Autodesk Inventor part; units mm, degrees
ref_plane "YZ Plane" through (0, 0, 0) normal (1, 0, 0) x (0, 1, 0)
ref_plane "XZ Plane" through (0, 0, 0) normal (0, 1, 0) x (-1, 0, 0)
ref_plane "XY Plane" through (0, 0, 0) normal (0, 0, 1) x (1, 0, 0)
sketch "Esboço1" plane through (0, 0, 0) normal (1, 0, 0) x (0, 1, 0)
  circle A0 centre (0, 0) radius 22.5
  dimension "d0" = 45
extrude "Extrusão1" add sketch "Esboço1" along normal blind 40
fillet "Arredondamento1" radius 10 1 edges at (0, -22.5, 0)
sketch "Esboço2" plane through (0, 0, 0) normal (-1, 0, 0) x (0, 0, 1)
  line L0 (0, 0) -> (0, -268) construction
  line L1 (-7.5, 0) -> (-7.5, -268)
  line L2 (7.5, -268) -> (7.5, 0)
  arc A0 (7.5, 0) -> (-7.5, 0) centre (0, 0) ccw
  arc A1 (-7.5, -268) -> (7.5, -268) centre (0, -268) ccw
  point P0 (0, -134)
  dimension "d5" = 15
extrude "Extrusão2" add sketch "Esboço2" along normal blind 30
fillet "Arredondamento2" radius 7 5 edges at (-30, -134, 7.5) (-30, 7.5, 0) (-30, -134, -7.5) (-30, -275.5, 0) (40, -22.5, 0)
sketch "Esboço3" plane through (0, -268, 7.5) normal (0, 0, 1) x (1, 0, 0)
  circle A0 centre (-11.5, 5) radius 6.25
  point P0 (0, 268)
extrude "Extrusão3" cut sketch "Esboço3" against normal blind 30
properties part number "braço"
Source: CAD feature listing. Evaluate the final solid. Frame: model axes, mm. A direction names the side the tool comes from. Round coordinates to 2 decimals unless told otherwise and drop trailing zeros. Loops run counter-clockwise (first coordinate to the right, second up) from the corner with the lowest first, then second, coordinate; pieces in that order, holes last.
1. Ray query, L1, parallel to Y at x = -11.5, z = 0.25; L2, parallel to X at y = -263, z = 4.75; L3, parallel to Z at x = -2, y = -250. Return the intervals inside material, ascending.
2. Section query B-B on x = -11.5. Output: boundary loops of the cut face in (y, z), and give its area (3 significant figures).
3. Section query D-D on x = 20. Output: boundary loops of the cut face in (y, z).
4. Access query for faces 5 (the flat face through (0, 9, 0)), 6 (the cylindrical face through (-28, -135.9, -5.4)). Directions: +Z, -Z, +X, -X, +Y, -Y. A direction counts if a zero-diameter tool reaches every point of the face in a straight line with its end or side. Return the directions, or none.
5. Section query C-C on y = -130. Output: boundary loops of the cut face in (x, z).
6. Section query A-A on y = -263. Output: boundary loops of the cut face in (x, z).
7. Contact query for flat-ended pins moving along their axis: pin 1 (5 mm diameter, centred on x = 7.5, z = 17.5, fed in from -Y); pin 2 (10 mm diameter, centred on y = -103.5, z = 12, fed in from +X); pin 3 (4 mm diameter, centred on x = -11.5, z = -1.5, fed in from +Y). Output: stop coordinate, or through.
8. Mould query, pull axis Y, two halves, no side actions, for faces 1 (the cylindrical face through (-12.855, -269.101, 0.105)), 2 (the cylindrical face through (21.339, 10.382, 19.961)), 3 (the cylindrical face through (-11.34, 7.5, -0.16)), 4 (the flat face through (-11, -136, 7.5)). Classes: released by +Y, released by -Y, zero draft, split by the parting line, or undercut.
Answers below:
1. L1: y = -275.5 to -269.25, -256.75 to 7.5
1. L2: x = -28.56 to -17.75, -5.25 to 0
1. L3: z = -7.5 to 7.5
2. outline: (-269.25, -7.4) - (-269.25, 7.4) arc R7.5 ccw to start; (-256.75, -7.5) - (0, -7.5) arc R7.5 ccw to (0, 7.5) - (-256.75, 7.5) - close
2. area: 4,010 mm2
3. outline: circle Ø45 at (0, 0)
4. face 5: -X, +Y
4. face 6: -Z, -X, +Y, -Y
5. outline: (-30, -0.5) arc R7 ccw to (-23, -7.5) - (0, -7.5) - (0, 7.5) - (-23, 7.5) arc R7 ccw to (-30, 0.5) - close
6. outline: (-30, -0.5) arc R7 ccw to (-23, -7.5) - (-17.75, -7.5) - (-17.75, 7.5) - (-23, 7.5) arc R7 ccw to (-30, 0.5) - close; (-5.25, -7.5) - (0, -7.5) - (0, 7.5) - (-5.25, 7.5) - close
7. pin 1: stops at y = -16.46
7. pin 2: stops at x = 0
7. pin 3: stops at y = 7.5
8. face 1: undercut
8. face 2: split by the parting line
8. face 3: released by +Y
8. face 4: zero draft
